For this review, take the finished solid that the model builds, in its own axes (mm). Round coordinates to 2 decimals unless told otherwise and drop trailing zeros. Loops run counter-clockwise (first coordinate to the right, second up) from the corner with the lowest first, then second, coordinate; pieces in that order, holes last. Notation, with made-up numbers: (23.5, 45.5) -> (34.5, 45.5) arc R10 cw to (34.5, 56.5) -> close; hole circle Ø2 at (-10, 43.5). An arc over 180 degrees is marked (long way). One line per question, with ' | ' between items. Start each with the question number.
1. Consider section A-A (x = 4.5). Count the separate pieces of the cut face and the enclosed holes in it, and give its area (3 significant figures).
2. Consider section B-B (z = -150). Write out the cut boundary in (x, y), and give its area (3 significant figures).
3. For pin 1 Ø5.5 at (y, z) = (22.225, -263.525) entering from -X; pin 2 Ø1.9 at (x, z) = (2.5, -165) entering from -Y, all flat-tipped, find the tip position at first contact; note any pin that passes through.
4. Wall thickness on line 1 along Z through (x, y) = (5.25, 39); line 2 along Y through (x, z) = (2.5, -241.3); line 3 along Y through (x, z) = (1, -203): over which ranges is each line inside the solid? List them lowest first.
```python
from build123d import *

# Parameters (mm, degrees)
BOSS_EXTRUDE1_DEPTH = 6.35
SKETCH3_R           = 3.96875
CUT_EXTRUDE1_DEPTH  = 7.35
SKETCH5_W           = 6.35
SKETCH5_H           = 12.7
CUT_EXTRUDE3_DEPTH  = 7.35
LPATTERN1_COUNT     = 16
LPATTERN1_PITCH     = 25.4
SKETCH6_W           = 6.35
SKETCH6_H           = 12.7
CUT_EXTRUDE4_DEPTH  = 7.35
LPATTERN2_COUNT     = 11
LPATTERN2_PITCH     = 25.4
SKETCH7_W           = 6.35
SKETCH7_H           = 12.7
SKETCH7_W_2         = 12.7
SKETCH7_H_2         = 6.35
CUT_EXTRUDE5_DEPTH  = 7.35
CUT_EXTRUDE6_DEPTH  = 7.35
LPATTERN3_COUNT     = 10
LPATTERN3_PITCH     = 25.4
SKETCH9_W           = 12.7
SKETCH9_H           = 6.35
CUT_EXTRUDE7_DEPTH  = 7.35
LPATTERN4_COUNT     = 8
LPATTERN4_PITCH     = 25.4
SKETCH10_R          = 3.175
CUT_EXTRUDE8_DEPTH  = 7.35
SKETCH11_R          = 3.96875
CUT_EXTRUDE9_DEPTH  = 7.35
SKETCH12_W          = 6.35
SKETCH12_H          = 12.7
CUT_EXTRUDE13_DEPTH = 7.35
CUT_EXTRUDE15_DEPTH = 7.35
CUT_EXTRUDE16_DEPTH = 7.35
SKETCH17_W          = 12.7
SKETCH17_H          = 6.35
CUT_EXTRUDE17_DEPTH = 7.35
LPATTERN5_COUNT     = 17
LPATTERN5_PITCH     = 25.4
LPATTERN6_COUNT     = 2
LPATTERN6_PITCH     = 120.65
SKETCH18_W          = 12.7
SKETCH18_H          = 6.35
CUT_EXTRUDE18_DEPTH = 7.35
LPATTERN7_COUNT     = 5
LPATTERN7_PITCH     = 25.4
CUT_EXTRUDE19_DEPTH = 7.35
SKETCH20_W          = 101.6
SKETCH20_H          = 57.15
CUT_EXTRUDE20_DEPTH = 7.35
CUT_EXTRUDE21_DEPTH = 7.35
CUT_EXTRUDE22_DEPTH = 7.35
BOSS_EXTRUDE4_DEPTH = 6.35
BOSS_EXTRUDE5_DEPTH = 6.35
SKETCH29_R          = 2.54
CUT_EXTRUDE23_DEPTH = 7.35
SKETCH30_R          = 1.75
CUT_EXTRUDE24_DEPTH = 7.35
FILLET2_R           = 6.35


with BuildPart() as part:
    # Sketch2 → Boss-Extrude1 (new body)
    with BuildSketch(Plane(origin=(0, 0, 0), x_dir=(0, 0, -1), z_dir=(1, 0, 0))):
        Polygon((0, 0), (0, 294.450076882), (215.9, 419.1), (431.8, 419.1), (431.8, 0), (241.3, 0), (241.3, 38.1), (127, 38.1), (127, 0), align=None)
    extrude(amount=BOSS_EXTRUDE1_DEPTH)

    # Sketch3 → Cut-Extrude1 (cut, through all)
    with BuildSketch(Plane(origin=(6.35, 0, 0), x_dir=(0, 0, -1), z_dir=(1, 0, 0))):
        with Locations((63.5, 38.1)):
            Circle(SKETCH3_R)
        with Locations((368.3, 38.1)):
            Circle(SKETCH3_R)
    extrude(amount=-CUT_EXTRUDE1_DEPTH, mode=Mode.SUBTRACT)

    # Sketch5 → Cut-Extrude3 (cut, through all)
    with BuildSketch(Plane(origin=(6.35, 0, 0), x_dir=(0, 0, -1), z_dir=(1, 0, 0))):
        with Locations((428.625, 19.05)):
            Rectangle(SKETCH5_W, SKETCH5_H)
    cut_extrude3 = extrude(amount=-CUT_EXTRUDE3_DEPTH, mode=Mode.SUBTRACT)

    # LPattern1: Cut-Extrude3 ×16
    with Locations(*[(0, i * LPATTERN1_PITCH, 0) for i in range(1, LPATTERN1_COUNT)]):
        add(cut_extrude3, mode=Mode.SUBTRACT)

    # Sketch6 → Cut-Extrude4 (cut, through all)
    with BuildSketch(Plane(origin=(6.35, 0, 0), x_dir=(0, 0, -1), z_dir=(1, 0, 0))):
        with Locations((3.175, 19.05)):
            Rectangle(SKETCH6_W, SKETCH6_H)
    cut_extrude4 = extrude(amount=-CUT_EXTRUDE4_DEPTH, mode=Mode.SUBTRACT)

    # LPattern2: Cut-Extrude4 ×11
    with Locations(*[(0, i * LPATTERN2_PITCH, 0) for i in range(1, LPATTERN2_COUNT)]):
        add(cut_extrude4, mode=Mode.SUBTRACT)

    # Sketch7 → Cut-Extrude5 (cut, through all)
    with BuildSketch(Plane(origin=(6.35, 0, 0), x_dir=(0, 0, -1), z_dir=(1, 0, 0))):
        with Locations((123.825, 19.05)):
            Rectangle(SKETCH7_W, SKETCH7_H)
        with Locations((133.35, 41.275)):
            Rectangle(SKETCH7_W_2, SKETCH7_H_2)
        with Locations((158.75, 41.275)):
            Rectangle(SKETCH7_W_2, SKETCH7_H_2)
        with Locations((184.15, 41.275)):
            Rectangle(SKETCH7_W_2, SKETCH7_H_2)
        with Locations((244.475, 19.05)):
            Rectangle(SKETCH7_W, SKETCH7_H)
        with Locations((209.55, 41.275)):
            Rectangle(SKETCH7_W_2, SKETCH7_H_2)
        with Locations((234.95, 41.275)):
            Rectangle(SKETCH7_W_2, SKETCH7_H_2)
    extrude(amount=-CUT_EXTRUDE5_DEPTH, mode=Mode.SUBTRACT)

    # Sketch8 → Cut-Extrude6 (cut, through all)
    with BuildSketch(Plane(origin=(6.35, 0, 0), x_dir=(0, 0, -1), z_dir=(1, 0, 0))):
        Polygon((201.93507044, 411.037344159), (212.933593068, 417.387344159), (216.108593068, 411.888082845), (205.11007044, 405.538082845), align=None)
    cut_extrude6 = extrude(amount=-CUT_EXTRUDE6_DEPTH, mode=Mode.SUBTRACT)

    # LPattern3: Cut-Extrude6 ×10
    with Locations(*[Vector(0, -0.5, 0.866025404) * (i * LPATTERN3_PITCH) for i in range(1, LPATTERN3_COUNT)]):
        add(cut_extrude6, mode=Mode.SUBTRACT)

    # Sketch9 → Cut-Extrude7 (cut, through all)
    with BuildSketch(Plane(origin=(6.35, 0, 0), x_dir=(0, 0, -1), z_dir=(1, 0, 0))):
        with Locations((412.75, 415.925)):
            Rectangle(SKETCH9_W, SKETCH9_H)
    cut_extrude7 = extrude(amount=-CUT_EXTRUDE7_DEPTH, mode=Mode.SUBTRACT)

    # LPattern4: Cut-Extrude7 ×8
    with Locations(*[(0, 0, i * LPATTERN4_PITCH) for i in range(1, LPATTERN4_COUNT)]):
        add(cut_extrude7, mode=Mode.SUBTRACT)

    # Sketch10 → Cut-Extrude8 (cut, through all)
    with BuildSketch(Plane(origin=(6.35, 0, 0), x_dir=(0, 0, -1), z_dir=(1, 0, 0))):
        with Locations((222.25, 273.05)):
            Circle(SKETCH10_R)
        with Locations((222.25, 57.15)):
            Circle(SKETCH10_R)
        with Locations((146.05, 57.15)):
            Circle(SKETCH10_R)
        with Locations((146.05, 273.05)):
            Circle(SKETCH10_R)
    extrude(amount=-CUT_EXTRUDE8_DEPTH, mode=Mode.SUBTRACT)

    # Sketch11 → Cut-Extrude9 (cut, through all)
    with BuildSketch(Plane(origin=(6.35, 0, 0), x_dir=(0, 0, -1), z_dir=(1, 0, 0))):
        with Locations((38.1, 260.35)):
            Circle(SKETCH11_R)
        with Locations((266.7, 260.35)):
            Circle(SKETCH11_R)
    extrude(amount=-CUT_EXTRUDE9_DEPTH, mode=Mode.SUBTRACT)

    # Sketch12 → Cut-Extrude13 (cut, through all)
    with BuildSketch(Plane(origin=(6.35, 0, 0), x_dir=(0, 0, -1), z_dir=(1, 0, 0))):
        with Locations((123.825, 44.45)):
            Rectangle(SKETCH12_W, SKETCH12_H)
        with Locations((123.825, 69.85)):
            Rectangle(SKETCH12_W, SKETCH12_H)
        with Locations((123.825, 95.25)):
            Rectangle(SKETCH12_W, SKETCH12_H)
        with Locations((123.825, 120.65)):
            Rectangle(SKETCH12_W, SKETCH12_H)
    cut_extrude13 = extrude(amount=-CUT_EXTRUDE13_DEPTH, mode=Mode.SUBTRACT)

    # Sketch14 → Cut-Extrude15 (cut, through all)
    with BuildSketch(Plane(origin=(6.35, 0, 0), x_dir=(0, 0, -1), z_dir=(1, 0, 0))):
        Polygon((36.957231019, 315.787344159), (47.955753647, 322.137344159), (51.130753647, 316.638082845), (40.132231019, 310.288082845), align=None)
        Polygon((80.951321531, 341.187344159), (91.949844159, 347.537344159), (95.124844159, 342.038082845), (84.126321531, 335.688082845), align=None)
    extrude(amount=-CUT_EXTRUDE15_DEPTH, mode=Mode.SUBTRACT)

    # Sketch15 → Cut-Extrude16 (cut, through all)
    with BuildSketch(Plane(origin=(6.35, 0, 0), x_dir=(0, 0, -1), z_dir=(1, 0, 0))):
        with BuildLine():
            Line((62.129276275, 322.988082845), (31.558579521, 305.338082845))
            ThreePointArc((31.558579521, 305.338082845), (51.535904978, 302.314952438), (62.501260575, 319.285333297))
            ThreePointArc((62.501260575, 319.285333297), (62.408031035, 321.146027155), (62.129276275, 322.988082845))
        make_face()
        with BuildLine():
            Line((103.698495657, 346.988082845), (73.127798903, 329.338082845))
            ThreePointArc((73.127798903, 329.338082845), (93.10512436, 326.314952438), (104.070479957, 343.285333297))
            ThreePointArc((104.070479957, 343.285333297), (103.977250417, 345.146027155), (103.698495657, 346.988082845))
        make_face()
    extrude(amount=-CUT_EXTRUDE16_DEPTH, mode=Mode.SUBTRACT)

    # Sketch17 → Cut-Extrude17 (cut, through all)
    with BuildSketch(Plane(origin=(6.35, 0, 0), x_dir=(0, 0, -1), z_dir=(1, 0, 0))):
        with Locations((25.4, 142.875)):
            Rectangle(SKETCH17_W, SKETCH17_H)
    cut_extrude17 = extrude(amount=-CUT_EXTRUDE17_DEPTH, mode=Mode.SUBTRACT)

    # LPattern5: Cut-Extrude17 ×17
    with Locations(*[(0, 0, -i * LPATTERN5_PITCH) for i in range(1, LPATTERN5_COUNT)]):
        add(cut_extrude17, mode=Mode.SUBTRACT)

    # LPattern6: Cut-Extrude13 ×2
    with Locations(*[(0, 0, -i * LPATTERN6_PITCH) for i in range(1, LPATTERN6_COUNT)]):
        add(cut_extrude13, mode=Mode.SUBTRACT)

    # Sketch18 → Cut-Extrude18 (cut, through all)
    with BuildSketch(Plane(origin=(6.35, 0, 0), x_dir=(0, 0, -1), z_dir=(1, 0, 0))):
        with Locations((133.35, 117.475)):
            Rectangle(SKETCH18_W, SKETCH18_H)
    cut_extrude18 = extrude(amount=-CUT_EXTRUDE18_DEPTH, mode=Mode.SUBTRACT)

    # LPattern7: Cut-Extrude18 ×5
    with Locations(*[(0, 0, -i * LPATTERN7_PITCH) for i in range(1, LPATTERN7_COUNT)]):
        add(cut_extrude18, mode=Mode.SUBTRACT)

    # Sketch19 → Cut-Extrude19 (cut, through all)
    with BuildSketch(Plane(origin=(6.35, 0, 0), x_dir=(0, 0, -1), z_dir=(1, 0, 0))):
        Polygon((25.4, 279.785380045), (222.705909488, 393.7), (406.4, 393.7), (406.4, 165.1), (25.4, 165.1), align=None)
    extrude(amount=-CUT_EXTRUDE19_DEPTH, mode=Mode.SUBTRACT)

    # Sketch20 → Cut-Extrude20 (cut, through all)
    with BuildSketch(Plane(origin=(6.35, 0, 0), x_dir=(0, 0, -1), z_dir=(1, 0, 0))):
        with Locations((184.15, 79.375)):
            Rectangle(SKETCH20_W, SKETCH20_H)
    extrude(amount=-CUT_EXTRUDE20_DEPTH, mode=Mode.SUBTRACT)

    # Sketch21 → Cut-Extrude21 (cut, through all)
    with BuildSketch(Plane(origin=(6.35, 0, 0), x_dir=(0, 0, -1), z_dir=(1, 0, 0))):
        Polygon((266.7, 25.4), (308.202954744, 25.4), (406.4, 82.094090512), (406.4, 133.35), (266.7, 133.35), align=None)
        Polygon((25.4, 133.35), (25.4, 82.094090512), (101.6, 38.1), (101.6, 133.35), align=None)
        Polygon((25.4, 38.1), (25.4, 25.4), (47.397045256, 25.4), align=None)
    extrude(amount=-CUT_EXTRUDE21_DEPTH, mode=Mode.SUBTRACT)

    # Sketch22 → Cut-Extrude22 (cut, through all)
    with BuildSketch(Plane(origin=(6.35, 0, 0), x_dir=(0, 0, -1), z_dir=(1, 0, 0))):
        Polygon((384.402954744, 25.4), (406.4, 38.1), (406.4, 25.4), align=None)
    extrude(amount=-CUT_EXTRUDE22_DEPTH, mode=Mode.SUBTRACT)

    # Sketch26 → Boss-Extrude4 (add, through all)
    with BuildSketch(Plane(origin=(6.35, 0, 0), x_dir=(0, 0, -1), z_dir=(1, 0, 0))):
        Polygon((266.7, 133.35), (266.7, 126.280871047), (278.944090512, 133.35), align=None)
        Polygon((89.355909488, 133.35), (101.6, 126.280871047), (101.6, 133.35), align=None)
        Polygon((266.7, 32.469128953), (278.944090512, 25.4), (266.7, 25.4), align=None)
        Polygon((133.35, 107.95), (133.35, 100.880871047), (145.594090512, 107.95), align=None)
        Polygon((234.95, 107.95), (222.705909488, 107.95), (234.95, 100.880871047), align=None)
        Polygon((133.35, 50.8), (145.594090512, 50.8), (133.35, 57.869128953), align=None)
        Polygon((234.95, 50.8), (222.705909488, 50.8), (234.95, 57.869128953), align=None)
    extrude(amount=-BOSS_EXTRUDE4_DEPTH)


with BuildPart() as body_2:
    # Sketch27 → Boss-Extrude5 (new body)
    with BuildSketch(Plane(origin=(6.35, 0, 0), x_dir=(0, 0, -1), z_dir=(1, 0, 0))):
        Polygon((12.7, 163.83), (12.7, 12.7), (114.3, 12.7), (114.3, 50.8), (254, 50.8), (254, 12.7), (419.1, 12.7), (419.1, 163.83), align=None)
    extrude(amount=-BOSS_EXTRUDE5_DEPTH)

    # Sketch29 → Cut-Extrude23 (cut, through all)
    with BuildSketch(Plane(origin=(6.35, 0, 0), x_dir=(0, 0, -1), z_dir=(1, 0, 0))):
        with Locations((38.1, 157.1625)):
            Circle(SKETCH29_R)
        with Locations((88.9, 157.1625)):
            Circle(SKETCH29_R)
        with Locations((139.7, 157.1625)):
            Circle(SKETCH29_R)
        with Locations((190.5, 157.1625)):
            Circle(SKETCH29_R)
        with Locations((241.3, 157.1625)):
            Circle(SKETCH29_R)
        with Locations((292.1, 157.1625)):
            Circle(SKETCH29_R)
        with Locations((342.9, 157.1625)):
            Circle(SKETCH29_R)
        with Locations((393.7, 157.1625)):
            Circle(SKETCH29_R)
    extrude(amount=-CUT_EXTRUDE23_DEPTH, mode=Mode.SUBTRACT)

    # Sketch30 → Cut-Extrude24 (cut, through all)
    with BuildSketch(Plane(origin=(6.35, 0, 0), x_dir=(0, 0, -1), z_dir=(1, 0, 0))):
        with Locations((22.225, 58.42)):
            Circle(SKETCH30_R)
        with Locations((104.775, 22.225)):
            Circle(SKETCH30_R)
        with Locations((263.525, 22.225)):
            Circle(SKETCH30_R)
        with Locations((409.575, 58.42)):
            Circle(SKETCH30_R)
    extrude(amount=-CUT_EXTRUDE24_DEPTH, mode=Mode.SUBTRACT)

    # Fillet2
    fillet2_edges = [body_2.edges().sort_by_distance(p)[0] for p in [
        (3.175, 163.83, -419.1),
        (3.175, 12.7, -419.1),
        (3.175, 12.7, -254),
        (3.175, 50.8, -254),
        (3.175, 50.8, -114.3),
        (3.175, 12.7, -114.3),
        (3.175, 12.7, -12.7),
        (3.175, 163.83, -12.7),
    ]]
    fillet(fillet2_edges, radius=FILLET2_R)


solid = body_2.part
```
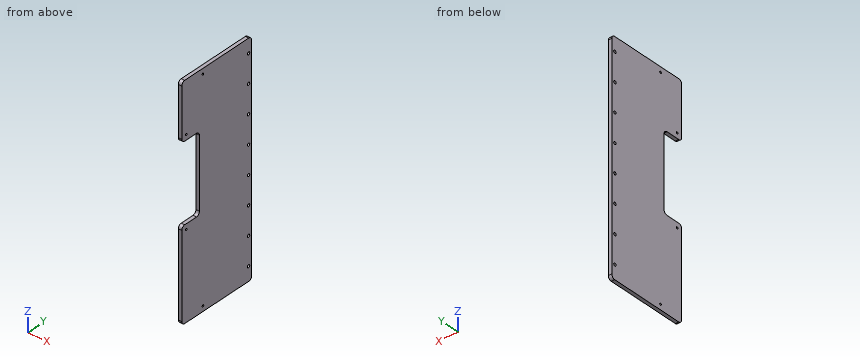
Answer block:
1) separate pieces: 1 | enclosed holes: 12 | area: 55,900 mm2
2) outline: (0, 50.8) -> (6.35, 50.8) -> (6.35, 163.83) -> (0, 163.83) -> close | area: 718 mm2
3) pin 1: stops at x = 0 | pin 2: stops at y = 50.8
4) line 1: z = -419.1 to -254, -114.3 to -12.7 | line 2: y = 50.8 to 154.62, 159.7 to 163.83 | line 3: y = 50.8 to 163.83
